Read the model definition and answer for the solid it produces. Units are mm, in the model's axes. A direction names the side the tool comes from. Round coordinates to 2 decimals unless told otherwise and drop trailing zeros. Write each loop counter-clockwise with the first axis right and the second up, starting at its lowest first coordinate (ties: lowest second). Pieces come first, ordered by that corner, then holes. Notation, with made-up numbers: (60, 48.5) - (95, 48.5) arc R27 ccw to (95, 84.5) - close; hole circle Ø11 at (-4.75, -8). An arc over 180 degrees is marked (long way). One line per item, written item: value. Start each with the question number.
(1) For faces 4 (the face through (-5, 55, -4)), 5 (the face through (-9.94, 1.97, -3.27)), 6 (the face through (15, 15, -5)), determine the directions among +Z, -Z, +X, -X, +Y, -Y from which every point of the face is accessible in a straight line to the end or side of a thin tool.
(2) A cutting plane is placed at B-B, the plane z = -10.5. Determine the outline of the cut face in (x, y), plus the area to 3 significant figures.
(3) A cutting plane is placed at A-A, the plane x = 7.5. Determine the outline of the cut face in (y, z).
(4) Flat-ended cylindrical pins translate along their axes: pin 1 Ø9 at (x, z) = (5.5, -11) entering from -Y; pin 2 Ø1.5 at (y, z) = (48.5, -11.5) entering from +X; pin 3 Ø8 at (y, z) = (68.5, 13) entering from -X; pin 4 Ø6.5 at (x, y) = (-1.5, 16.5) entering from -Z. Find the tip coordinate at first contact, or state that the pin passes through.
(5) A cutting plane is placed at D-D, the plane z = 13. Determine the outline of the cut face in (x, y), plus the area to 3 significant figures.
(6) Find the intervals of material crossed by L1, parallel to X at y = 24, z = -11; L2, parallel to Y at x = -12.5, z = -1; L3, parallel to X at y = 1.2, z = -2, in increasing order.
(7) A cutting plane is placed at C-C, the plane x = -3. Determine the outline of the cut face in (y, z), plus the area to 3 significant figures.
(8) The mould has two halves that part along Z. Classify faces 1 (the face through (0, 15, 10)), 2 (the face through (0.07, 39.52, -1.34)), 3 (the face through (-20, 15, 0)): +Z half, -Z half, draft (parallel to the pull), parting line (faces both ways), or undercut.
from build123d import *

# Parameters (mm, degrees)
SKETCH1_W           = 40
SKETCH1_H           = 40
SKETCH1_W_2         = 20
SKETCH1_H_2         = 20
BOSS_EXTRUDE1_DEPTH = 30
SKETCH4_W           = 10
SKETCH4_H           = 40
BOSS_EXTRUDE3_DEPTH = 50
SKETCH5_R           = 2.5
CUT_EXTRUDE4_DEPTH  = 87.168439698
LPATTERN1_COUNT     = 6
LPATTERN1_PITCH     = 7.5
FILLET1_R           = 15
SKETCH6_W           = 30
SKETCH6_H           = 22
CUT_EXTRUDE5_DEPTH  = 30
CUT_EXTRUDE6_REACH  = 86.853
SKETCH7_R           = 2.75


with BuildPart() as part:
    # Sketch1 → Boss-Extrude1 (new body)
    # profile 1 of 2: a face of its own
    with BuildSketch(Plane(origin=(0, 0, 0), x_dir=(1, 0, 0), z_dir=(0, 1, 0))):
        Rectangle(SKETCH1_W, SKETCH1_H)
        Rectangle(SKETCH1_W_2, SKETCH1_H_2, mode=Mode.SUBTRACT)
    # profile 2 of 2: a face of its own
    with BuildSketch(Plane(origin=(0, 0, 0), x_dir=(1, 0, 0), z_dir=(0, 1, 0))):
        Rectangle(SKETCH1_W_2, SKETCH1_H_2)
    extrude(amount=BOSS_EXTRUDE1_DEPTH)

    # Sketch4 → Boss-Extrude3 (add)
    with BuildSketch(Plane(origin=(0, 30, 0), x_dir=(1, 0, 0), z_dir=(0, 1, 0))):
        Rectangle(SKETCH4_W, SKETCH4_H)
    extrude(amount=BOSS_EXTRUDE3_DEPTH)

    # Sketch5 → Cut-Extrude4 (cut, through all)
    with BuildSketch(Plane(origin=(5, 0, 0), x_dir=(0, 0, -1), z_dir=(1, 0, 0))):
        with Locations((0, 37.407153601)):
            Circle(SKETCH5_R)
    cut_extrude4 = extrude(amount=-CUT_EXTRUDE4_DEPTH, mode=Mode.SUBTRACT)

    # LPattern1: Cut-Extrude4 ×6
    with Locations(*[(0, i * LPATTERN1_PITCH, 0) for i in range(1, LPATTERN1_COUNT)]):
        add(cut_extrude4, mode=Mode.SUBTRACT)

    # Fillet1
    fillet1_edges = [part.edges().sort_by_distance(p)[0] for p in [
        (0, 80, -20),
        (0, 80, 20),
    ]]
    fillet(fillet1_edges, radius=FILLET1_R)

    # Sketch6 → Cut-Extrude5 (cut)
    with BuildSketch(Plane(origin=(0, 0, -20), x_dir=(-1, 0, 0), z_dir=(0, 0, -1))):
        with Locations((0, 15)):
            Rectangle(SKETCH6_W, SKETCH6_H)
    extrude(amount=-CUT_EXTRUDE5_DEPTH, mode=Mode.SUBTRACT)

    # Sketch7 → Cut-Extrude6 (cut, up to next)
    with BuildSketch(Plane.XZ, mode=Mode.PRIVATE) as cut_extrude6_sk1:
        with Locations(Location((-7.5, -2, 0), (0, 0, 270))):
            Circle(SKETCH7_R)
    cut_extrude6_tool1 = extrude(cut_extrude6_sk1.sketch, amount=-CUT_EXTRUDE6_REACH, mode=Mode.PRIVATE) & part.part
    # Sketch7 → Cut-Extrude6 (cut, up to next)
    with BuildSketch(Plane.XZ, mode=Mode.PRIVATE) as cut_extrude6_sk2:
        with Locations(Location((7.5, -2, 0), (0, 0, 270))):
            Circle(SKETCH7_R)
    cut_extrude6_tool2 = extrude(cut_extrude6_sk2.sketch, amount=-CUT_EXTRUDE6_REACH, mode=Mode.PRIVATE) & part.part
    add(cut_extrude6_tool1.solids().sort_by_distance((-7.5, 0, -2))[0], mode=Mode.SUBTRACT)
    add(cut_extrude6_tool2.solids().sort_by_distance((7.5, 0, -2))[0], mode=Mode.SUBTRACT)


solid = part.part
Here are the results:
1. face 4: +Z, -Z, -X, +Y
1. face 5: -Y
1. face 6: -Z
2. outline: (-20, 0) - (20, 0) - (20, 30) - (5, 30) - (5, 78.96) - (-5, 78.96) - (-5, 30) - (-20, 30) - close; hole (-15, 4) - (15, 4) - (15, 26) - (-15, 26) - close
2. area: 1,030 mm²
3. outline: (0, -20) - (4, -20) - (4, -4.75) - (0, -4.75) - close; (0, 0.75) - (4, 0.75) - (4, 10) - (26, 10) - (26, -20) - (30, -20) - (30, 20) - (0, 20) - close
4. pin 1: y = 0
4. pin 2: x = 5
4. pin 3: x = -5
4. pin 4: z = 10
5. outline: (-20, 0) - (20, 0) - (20, 30) - (5, 30) - (5, 77.69) - (-5, 77.69) - (-5, 30) - (-20, 30) - close
5. area: 1,680 mm²
6. L1: -20 to -15, 15 to 20
6. L2: 0 to 4, 26 to 30
6. L3: -20 to -10.25, -4.75 to 4.75, 10.25 to 20
7. outline: (0, -20) - (4, -20) - (4, 10) - (26, 10) - (26, -20) - (65, -20) arc R15 ccw to (80, -5) - (80, 5) arc R15 ccw to (65, 20) - (0, 20) - close; hole circle Ø5 at (37.41, 0); hole circle Ø5 at (44.91, 0); hole circle Ø5 at (52.41, 0); hole circle Ø5 at (59.91, 0); hole circle Ø5 at (67.41, 0); hole circle Ø5 at (74.91, 0)
7. area: 2,330 mm²
8. face 1: -Z half
8. face 2: undercut
8. face 3: draft
